The listing builds one solid part. Answer for the finished solid, in the listing's coordinates (mm). Coordinates: 2 decimals unless noted, no trailing zeros. Order: outer loops, then holes, each group sorted by start corner. A loop starts at its lowest first (then second) coordinate and runs counter-clockwise, first axis right, second up. Notation, with made-up numbers: (27, 23.5) -> (86, 23.5) arc R21 ccw to (86, 48.5) -> close; hole circle Ø7 at (5.25, 63.5). An arc over 180 degrees is marked (long way). Return JSON: item names as keys, results as strings.
from build123d import *

# Parameters (mm, degrees)
F0_W     = 300
F0_H     = 300
F0_W_2   = 134
F0_H_2   = 134
F1_DEPTH = 4
F2_R     = 1.99999
F3_SIZE  = 3.99999


# Not quite as in the source:
# - a fillet or chamfer is up to 0.001 mm smaller than in the source, because OpenCascade refuses the exact size


with BuildPart() as f1:
    # F0 (on Front) → F1 (new body)
    with BuildSketch(Plane.XZ):
        Rectangle(F0_W, F0_H)
        Rectangle(F0_W_2, F0_H_2, mode=Mode.SUBTRACT)
    extrude(amount=F1_DEPTH)

    # F2 (radius 2 in the source; OpenCascade refuses exactly that, so slightly less here)
    f2_edges = [f1.edges().sort_by_distance(p)[0] for p in [
        (0, -4, 150),
        (-150, -4, 0),
        (150, -4, 0),
        (0, -4, -150),
        (-150, 0, 0),
        (-150, -2, 150),
        (-150, -2, -150),
        (0, 0, -150),
        (150, 0, 0),
        (0, 0, 150),
        (150, -2, 150),
        (150, -2, -150),
    ]]
    fillet(f2_edges, radius=F2_R)

    # F3 (size 4 in the source; OpenCascade refuses exactly that, so slightly less here)
    f3_edges = [f1.edges().sort_by_distance(p)[0] for p in [
        (0, -4, 67),
        (67, -4, 0),
        (0, -4, -67),
        (-67, -4, 0),
    ]]
    chamfer(f3_edges, length=F3_SIZE)


solid = f1.part
1. This flat-tipped pin is pushed along its axis until it touches: pin 1 Ø1.5 at (x, y) = (-48, -1) entering from +Z. Where does it stop, or does it pass through?
Answer block:
{"pin 1": "stops at z = 149.98"}
2. The part is cut by section C-C on y = -1.1. Give the vertices of the cut face in (x, z), and give its area (3 significant figures).
Answer block:
{"outline": "(-149.79, -148) arc R1.79 ccw to (-148, -149.79) -> (148, -149.79) arc R1.79 ccw to (149.79, -148) -> (149.79, 148) arc R1.79 ccw to (148, 149.79) -> (-148, 149.79) arc R1.79 ccw to (-149.79, 148) -> close; hole (-68.1, -68.1) -> (68.1, -68.1) -> (68.1, 68.1) -> (-68.1, 68.1) -> close", "area": "71,200 mm2"}
3. Consider line 1 (Z direction, x = -116, y = -2.15); line 2 (Z direction, x = -103, y = -1.55); line 3 (X direction, y = -0.2, z = -31). Determine where each line is inside the solid, lowest interval first. Write a range as from..to.
Answer block:
{"line 1": "z = -149.99..149.99", "line 2": "z = -149.95..149.95", "line 3": "x = -148.87..-67.2, 67.2..148.87"}
